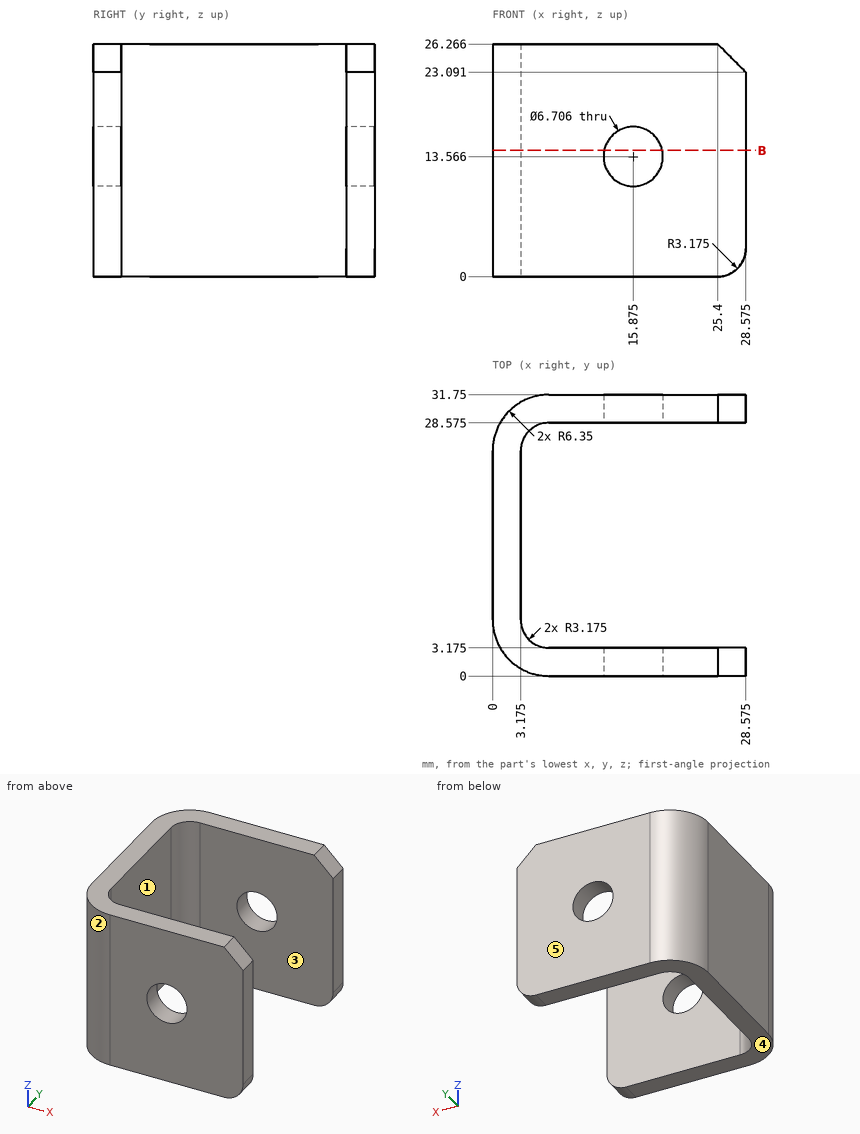
Can you work these out from the drawing? Everything is in mm from the part's minimum corner. A direction names the side the tool comes from. Give positions to 0.01 mm unless a question says otherwise; leave off trailing zeros. Write each question's results on one line, items separated by ' | '. Start each with the question number.
Q1. I'm going to push flat-ended pins straight in: pin 1 Ø5 at (x, z) = (14.5, 21) entering from -Y; pin 2 Ø10 at (x, y) = (23, 9) entering from -Z; pin 3 Ø8 at (y, z) = (8, 17) entering from +X (1 decimal); pin 4 Ø4 at (y, z) = (14.5, 22.5) entering from +X (3 decimals). Where does each tip first touch, or does it pass through?
Q2. I need wall thicknesses on probe 1 along X at (y, z) = (21, 1.5) (1 decimal); probe 2 along X at (y, z) = (30, 1) (1 decimal). Which ranges of each line are inside material? Lowest first, please.
Q3. We'd pull the mould along Y, two halves only. Please class the marked faces 3, 4 and 5: +Y half, -Y half, draft (parallel to the pull), parting line (faces both ways), or undercut.
Q4. Which directions (+Z, -Z, +X, -X, +Y, -Y) give clear straight access to the entire face, cutting with the end or side of a thin tool? Please do the marked faces 1 and 2.
Q5. Suppose I cut it at B-B, the plane z = 14.25. State how many separate pieces and enclosed holes the cut face has.
Outcome:
1) pin 1: y = 0 | pin 2: through | pin 3: x = 4.2 | pin 4: x = 3.175
2) probe 1: 0 to 3.2 | probe 2: 2 to 27.7
3) face 3: undercut | face 4: draft | face 5: +Y half
4) face 1: +Z, -Z, +X | face 2: +Z, -Z, -X, -Y
5) separate pieces: 3 | enclosed holes: 0
